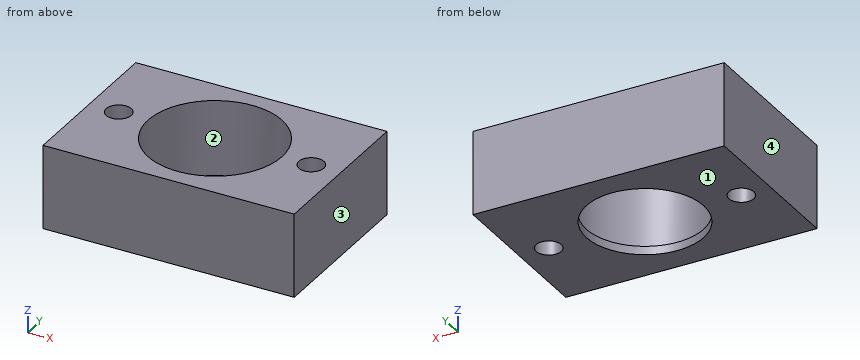
from build123d import *

# Parameters (mm, degrees)
SKETCH1_W           = 30
SKETCH1_H           = 20
SKETCH1_R           = 1.5
SKETCH1_R_2         = 8
BOSS_EXTRUDE1_DEPTH = 10
SKETCH1_3_R         = 8
SKETCH1_3_R_2       = 7
BOSS_EXTRUDE2_DEPTH = 1


with BuildPart() as part:
    # Sketch1 → Boss-Extrude1 (new body)
    with BuildSketch(Plane.XY):
        with Locations((7.259887006, 7.881355932)):
            Rectangle(SKETCH1_W, SKETCH1_H)
        with Locations((18.759887006, 7.881355932)):
            Circle(SKETCH1_R, mode=Mode.SUBTRACT)
        with Locations((-4.240112994, 7.881355932)):
            Circle(SKETCH1_R, mode=Mode.SUBTRACT)
        with Locations((7.259887006, 7.881355932)):
            Circle(SKETCH1_R_2, mode=Mode.SUBTRACT)
    extrude(amount=BOSS_EXTRUDE1_DEPTH)

    # Sketch1<3> → Boss-Extrude2 (add)
    with BuildSketch(Plane.XY):
        with Locations((7.259887006, 7.881355932)):
            Circle(SKETCH1_3_R)
        with Locations((7.259887006, 7.881355932)):
            Circle(SKETCH1_3_R_2, mode=Mode.SUBTRACT)
    extrude(amount=BOSS_EXTRUDE2_DEPTH)


solid = part.part
For this review, take the finished solid that the model builds, in its own axes (mm). Face numbers are marked on the shaded views. Round coordinates to 2 decimals unless told otherwise and drop trailing zeros. Loops run counter-clockwise (first coordinate to the right, second up) from the corner with the lowest first, then second, coordinate; pieces in that order, holes last. Notation, with made-up numbers: (-21.5, 10.25) - (17.5, 10.25) arc R25 ccw to (17.5, 46.25) - close; hole circle Ø3 at (41, 55.5). An arc over 180 degrees is marked (long way). One line per item, written item: value. Start each with the question number.
Item 1: Take a section at C-C (z = 3.75). Give the boundary of the cut face in (x, y).
Item 2: Take a section at D-D (y = 8.25). Give the boundary of the cut face in (x, z), plus the area to 3 significant figures.
Item 3: Take a section at B-B (y = 5.25). Give the boundary of the cut face in (x, z), plus the area to 3 significant figures.
Item 4: The part is to be moulded in two halves that separate along X. For the marked faces 1, 2, 3 and 4, say which applies: +X half, -X half, draft (parallel to the pull), parting line (faces both ways), or undercut.
Item 5: Take a section at A-A (x = 6.25). Give the boundary of the cut face in (y, z).
Item 6: For L1, parallel to X at y = 8, z = 9.5; L2, parallel to X at y = 7, z = 3; L3, parallel to X at y = 4, z = 3.25, list the stretches that pass through material, from the lowest coordinate up.
Item 7: Clearance check with flat-ended pins moving along their axes: pin 1 Ø1.5 at (x, y) = (4.5, 4) entering from -Z; pin 2 Ø4 at (x, y) = (3.5, 11.5) entering from +Z. State where each tip first meets the part, or that it passes through.
Answer below:
1. outline: (-7.74, -2.12) - (22.26, -2.12) - (22.26, 17.88) - (-7.74, 17.88) - close; hole circle Ø3 at (-4.24, 7.88); hole circle Ø16 at (7.26, 7.88); hole circle Ø3 at (18.76, 7.88)
2. outline: (-7.74, 0) - (-5.69, 0) - (-5.69, 10) - (-7.74, 10) - close; (-2.79, 0) - (0.27, 0) - (0.27, 1) - (-0.73, 1) - (-0.73, 10) - (-2.79, 10) - close; (14.25, 0) - (17.31, 0) - (17.31, 10) - (15.25, 10) - (15.25, 1) - (14.25, 1) - close; (20.21, 0) - (22.26, 0) - (22.26, 10) - (20.21, 10) - close
2. area: 84.0 mm2
3. outline: (-7.74, 0) - (0.77, 0) - (0.77, 1) - (-0.29, 1) - (-0.29, 10) - (-7.74, 10) - close; (13.75, 0) - (22.26, 0) - (22.26, 10) - (14.81, 10) - (14.81, 1) - (13.75, 1) - close
3. area: 151 mm2
4. face 1: draft
4. face 2: undercut
4. face 3: +X half
4. face 4: -X half
5. outline: (-2.12, 0) - (0.95, 0) - (0.95, 1) - (-0.05, 1) - (-0.05, 10) - (-2.12, 10) - close; (14.81, 0) - (17.88, 0) - (17.88, 10) - (15.82, 10) - (15.82, 1) - (14.81, 1) - close
6. L1: x = -7.74 to -5.74, -2.74 to -0.74, 15.26 to 17.26, 20.26 to 22.26
6. L2: x = -7.74 to -5.45, -3.03 to -0.69, 15.21 to 17.55, 19.97 to 22.26
6. L3: x = -7.74 to 0.26, 14.26 to 22.26
7. pin 1: passes through
7. pin 2: stops at z = 1
